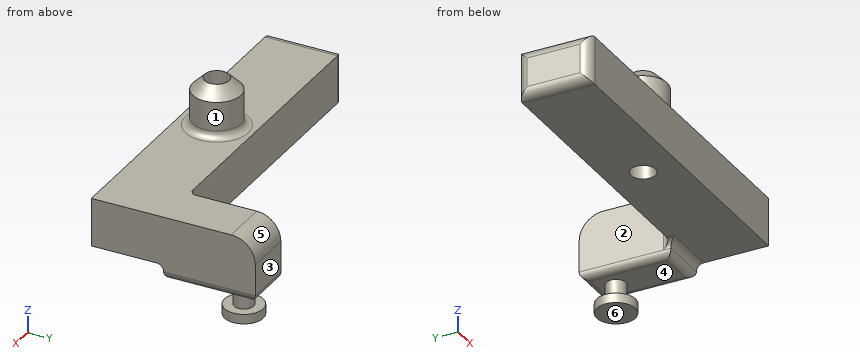
```python
from build123d import *

# Parameters (mm, degrees)
SKETCH1_W                = 70
SKETCH1_H                = 15
SKETCH1_R                = 2.55
BOSS_EXTRUDE1_DEPTH      = 10
BOSS_EXTRUDE5_DEPTH      = 3
BOSS_EXTRUDE5_DEPTH_BACK = 10
SKETCH5_W                = 10
SKETCH5_H                = 19
FILLET1_R                = 2
SKETCH3_R                = 2
BOSS_EXTRUDE6_DEPTH      = 4
SKETCH6_R                = 4
BOSS_EXTRUDE7_DEPTH      = 2
FILLET4_R                = 5
FILLET3_R                = 1.5
FILLET9_R                = 1.5
SKETCH9_R                = 2.55
CUT_EXTRUDE1_DEPTH       = 10
FILLET10_R               = 1.5


# Some blends are built 0.0001 mm under size
with BuildPart() as part:
    # Sketch1 → Boss-Extrude1 (new body)
    with BuildSketch(Plane.XY):
        Rectangle(SKETCH1_W, SKETCH1_H)
        Circle(SKETCH1_R, mode=Mode.SUBTRACT)
    extrude(amount=BOSS_EXTRUDE1_DEPTH)

    # Fillet1
    fillet1_edges = [part.edges().sort_by_distance(p)[0] for p in [
        (-35, 0, 10),
        (-35, 0, 0),
        (-35, 7.5, 5),
        (-35, -7.5, 5),
    ]]
    fillet(fillet1_edges, radius=FILLET1_R)


with BuildPart() as body_2:
    # Sketch5 → Boss-Extrude5 (new, two sides: drawn at the far end of the back side and taken through both)
    with BuildSketch(Plane(origin=(0, 0, 0), x_dir=(-1, 0, 0), z_dir=(0, 0, -1)).offset(-BOSS_EXTRUDE5_DEPTH_BACK)):
        with Locations((-30, 17)):
            Rectangle(SKETCH5_W, SKETCH5_H)
    extrude(amount=BOSS_EXTRUDE5_DEPTH + BOSS_EXTRUDE5_DEPTH_BACK)

    # Fillet4
    fillet4_edges = [body_2.edges().sort_by_distance(p)[0] for p in [
        (30, 26.5, 10),
    ]]
    fillet(fillet4_edges, radius=FILLET4_R)


with BuildPart() as body_3:
    # Sketch3 → Boss-Extrude6 (new body)
    with BuildSketch(Plane(origin=(-35, 0, -3), x_dir=(-1, 0, 0), z_dir=(0, 0, -1))):
        with Locations((-65, 21.5)):
            Circle(SKETCH3_R)
    extrude(amount=BOSS_EXTRUDE6_DEPTH)


with BuildPart() as body_4:
    # Sketch6 → Boss-Extrude7 (new body)
    with BuildSketch(Plane(origin=(0, 0, -7), x_dir=(-1, 0, 0), z_dir=(0, 0, -1))):
        with Locations((-30, 21.5)):
            Circle(SKETCH6_R)
    extrude(amount=BOSS_EXTRUDE7_DEPTH)


with BuildPart() as body_3_1:
    add(body_3.part)

    # Combine1: union body 2, body 4, part
    add(body_2.part)
    add(body_4.part)
    add(part.part)

    # Fillet3
    # the kernel refuses this fillet: 1.5 mm, written as the material it adds along each edge
    with BuildSketch(Plane(origin=(35, 7.5, 0), x_dir=(0, 0, -1), z_dir=(-1, 0, 0))) as fillet3_piece_1:
        with BuildLine():
            CenterArc((FILLET3_R, FILLET3_R), FILLET3_R, 180, 90)
            Line((0, FILLET3_R), (0, 0))
            Line((0, 0), (FILLET3_R, 0))
        make_face()
    extrude(amount=10)
    # the kernel refuses this fillet: 1.5 mm, written as the material it takes off along each edge
    with BuildSketch(Plane(origin=(21.25, 7.5, -3), x_dir=(0, 1, 0), z_dir=(1, 0, 0))) as fillet3_2_piece_1:
        with BuildLine():
            CenterArc((FILLET3_R, FILLET3_R), FILLET3_R, 180, 90)
            Line((0, FILLET3_R), (0, 0))
            Line((0, 0), (FILLET3_R, 0))
        make_face()
    extrude(amount=17.5, mode=Mode.SUBTRACT)
    with BuildSketch(Plane(origin=(25, 30.25, -3), x_dir=(0, 0, 1), z_dir=(0, -1, 0))) as fillet3_2_piece_2:
        with BuildLine():
            CenterArc((FILLET3_R, -FILLET3_R), FILLET3_R, 90, 90)
            Line((0, -FILLET3_R), (0, 0))
            Line((0, 0), (FILLET3_R, 0))
        make_face()
    extrude(amount=26.5, mode=Mode.SUBTRACT)
    with BuildSketch(Plane(origin=(38.75, 26.5, -3), x_dir=(0, 0, 1), z_dir=(-1, 0, 0))) as fillet3_2_piece_3:
        with BuildLine():
            CenterArc((FILLET3_R, -FILLET3_R), FILLET3_R, 90, 90)
            Line((0, -FILLET3_R), (0, 0))
            Line((0, 0), (FILLET3_R, 0))
        make_face()
    extrude(amount=17.5, mode=Mode.SUBTRACT)
    with BuildSketch(Plane(origin=(35, 3.75, -3), x_dir=(-1, 0, 0), z_dir=(0, 1, 0))) as fillet3_2_piece_4:
        with BuildLine():
            CenterArc((FILLET3_R, FILLET3_R), FILLET3_R, 180, 90)
            Line((0, FILLET3_R), (0, 0))
            Line((0, 0), (FILLET3_R, 0))
        make_face()
    extrude(amount=26.5, mode=Mode.SUBTRACT)

    # Fillet9
    fillet9_edges = [body_3_1.edges().sort_by_distance(p)[0] for p in [
        (25, 6.75, 0),
        (25, 7.5, 5),
    ]]
    fillet(fillet9_edges, radius=FILLET9_R - 0.0001)  # a hair under: the kernel refuses the full size

    # Sketch8 → Revolve1 (revolve)
    with BuildSketch(Plane(origin=(0, 0, 0), x_dir=(0, 0, -1), z_dir=(1, 0, 0))):
        Polygon((-10, 0), (-20, 0), (-20, 2.5), (-17.5, 5), (-10, 5), align=None)
    revolve(axis=Axis((0, 0, 10), (0, 0, 1)))

    # Sketch9 → Cut-Extrude1 (cut)
    with BuildSketch(Plane(origin=(0, 0, 10), x_dir=(-1, 0, 0), z_dir=(0, 0, -1))):
        with Locations(Location((0, 0, 0), (0, 0, 90))):
            Circle(SKETCH9_R)
    extrude(amount=-CUT_EXTRUDE1_DEPTH, mode=Mode.SUBTRACT)

    # Fillet10
    fillet10_edges = [body_3_1.edges().sort_by_distance(p)[0] for p in [
        (0, -5, 10),
    ]]
    fillet(fillet10_edges, radius=FILLET10_R)


solid = body_3_1.part
```
Check sheet for the modelled part. Datum: model origin and axes. Units: mm. Face numbers are marked on the shaded views. A direction names the side the tool comes from. Round coordinates to 2 decimals unless told otherwise and drop trailing zeros. Write each loop counter-clockwise with the first axis right and the second up, starting at its lowest first coordinate (ties: lowest second). Pieces come first, ordered by that corner, then holes. Notation, with made-up numbers: M 77,83.5 L 89,83.5 A17 ccw 89,107.5 Z; hole C -27.75,-31.5 d11. An arc over 180 degrees is marked long. Write item = value, one per line. Start each with the question number.
1. Release check for a two-part mould opening along Z. For the marked faces 4, 5 and 6 record: pulls with the +Z half, pulls with the -Z half, needs draft (parallel to the pull), parting line crosses it, or undercut.
2. Section check A-A, the plane x = 0. Record the cut outline in (y, z), then the cut area to 3 significant figures.
3. Tool access check on the marked faces 1, 2 and 3. Record the directions out of +Z, -Z, +X, -X, +Y, -Y that give a thin tool (end or side, any length) a straight path to the whole face; none if there is none.
4. Section check D-D, the plane z = 1.25. Record the cut outline in (x, y), then the cut area to 3 significant figures.
5. Gauge pin test, flat ends, axial feed: pin 1 (4 mm diameter, centred on x = -15, y = 10.5, fed in from -Z); pin 2 (2 mm diameter, centred on y = 10, z = -2, fed in from -X); pin 3 (16.5 mm diameter, centred on x = -2, y = -1.5, fed in from -Z); pin 4 (8 mm diameter, centred on x = -3.5, z = 5.5, fed in from +Y). Record the tip position at first contact, or that the pin passes through.
6. Section check C-C, the plane x = 30. Record the cut outline in (y, z).
7. Section check B-B, the plane y = 11. Record the cut outline in (x, z), then the cut area to 3 significant figures.
8. Scan lines: line 1 (Y direction, x = 0, z = 17); line 2 (X direction, y = 0, z = 6.75). Record each from-to range of solid material in increasing order. Write a range as [from, to].
Results found:
q1.face_4 = undercut
q1.face_5 = pulls with the +Z half
q1.face_6 = pulls with the -Z half
q2.outline = M -7.5,0 L -2.55,0 L -2.55,19.95 L -5,17.5 L -5,11.5 A1.5 cw -6.5,10 L -7.5,10 Z; M 2.55,0 L 7.5,0 L 7.5,10 L 6.5,10 A1.5 cw 5,11.5 L 5,17.5 L 2.55,19.95 Z
q2.area = 143 mm^2
q3.face_1 = +Z
q3.face_2 = +Z, -Z, -X, +Y
q3.face_3 = +Z, -Z, +X, -X, +Y
q4.outline = M -34.85,-6.25 A2 ccw -33,-7.5 L 35,-7.5 L 35,26.5 L 25,26.5 L 25,9 A1.5 cw 23.5,7.5 L -33,7.5 A2 ccw -34.85,6.25 Z; hole C 0,0 d5.1
q4.area = 1,220 mm^2
q5.pin_1 = through
q5.pin_2 = 25
q5.pin_3 = 0
q5.pin_4 = 7.5
q6.outline = M -7.5,0 L 6,0 A1.5 cw 7.5,-1.5 A1.5 ccw 9,-3 L 19.5,-3 L 19.5,-7 L 17.5,-7 L 17.5,-9 L 25.5,-9 L 25.5,-7 L 23.5,-7 L 23.5,-3 L 25,-3 A1.5 ccw 26.5,-1.5 L 26.5,5 A5 ccw 21.5,10 L -7.5,10 Z
q7.outline = M 25,-1.5 A1.5 ccw 26.5,-3 L 33.5,-3 A1.5 ccw 35,-1.5 L 35,10 L 25,10 Z
q7.area = 129 mm^2
q8.line_1 = [-5, -2.55], [2.55, 5]
q8.line_2 = [-35, -2.55], [2.55, 35]
